Autodesk Inventor part; units mm, degrees
ref_plane "YZ Plane" through (0, 0, 0) normal (1, 0, 0) x (0, 1, 0)
ref_plane "XZ Plane" through (0, 0, 0) normal (0, 1, 0) x (-1, 0, 0)
ref_plane "XY Plane" through (0, 0, 0) normal (0, 0, 1) x (1, 0, 0)
sketch "Skizze1" plane through (0, 0, 0) normal (0, 1, 0) x (-1, 0, 0)
  line L0 (87.5, -100) -> (-87.5, -100)
  line L1 (-87.5, -100) -> (-87.5, 100)
  line L2 (-87.5, 100) -> (87.5, 100)
  line L3 (87.5, 100) -> (87.5, -100)
  line L4 (0, -140) -> (0, 140)
  line L5 (122.5, 0) -> (-122.5, 0)
  point P0 (0, 0)
  dimension "d0" = 175
  dimension "d1" = 200
extrude "Extrusion1" add sketch "Skizze1" along normal blind 2
sketch "Skizze2" plane through (0, 2, 0) normal (0, 1, 0) x (1, 0, 0)
  circle A0 centre (54.5, 95) radius 1.6
  circle A1 centre (-82.5, 95) radius 1.6
  line L0 (0, 140) -> (0, -140)
  line L1 (122.5, 0) -> (-122.5, 0)
  line L2 (87.5, 100) -> (-87.5, 100)
  circle A2 centre (54.5, -95) radius 1.6
  circle A3 centre (-82.5, -95) radius 1.6
  line L3 (-87.5, 100) -> (-87.5, -100)
  line L4 (87.5, -100) -> (87.5, 100)
  point P0 (0, 0)
  dimension "d4" = 3.2
  dimension "d5" = 3.2
  dimension "d7" = 5
  dimension "d9" = 5
  dimension "d55" = 5
  dimension "d56" = 33
extrude "Extrusion2" cut sketch "Skizze2" against normal up to surface (2 mm away) contours A0 | A1 | A2 | A3
sketch "Skizze3" plane through (0, 2, 0) normal (0, 1, 0) x (1, 0, 0)
  line L0 (0, 140) -> (0, -140)
  line L1 (122.5, 0) -> (-122.5, 0)
  line L2 (-87.5, -100) -> (87.5, -100)
  line L3 (-87.5, 100) -> (-87.5, -100)
  circle A0 centre (64.5, -89.5) radius 1.6
  line L4 (87.5, -100) -> (87.5, 100)
  circle A1 centre (64.5, -25.5) radius 1.6
  circle A2 centre (64.5, 25.5) radius 1.6
  line L5 (87.5, 100) -> (-87.5, 100)
  circle A3 centre (64.5, 89.5) radius 1.6
  circle A4 centre (27.5, -23) radius 1.6
  circle A5 centre (27.5, 23) radius 1.6
  point P0 (0, 0)
  dimension "d35" = 3.2
  dimension "d36" = 10.5
  dimension "d37" = 23
  dimension "d38" = 3.2
  dimension "d39" = 74.5
  dimension "d40" = 23
  dimension "d41" = 3.2
  dimension "d42" = 23
  dimension "d43" = 74.5
  dimension "d44" = 3.2
  dimension "d45" = 23
  dimension "d46" = 10.5
  dimension "d47" = 3.2
  dimension "d48" = 60
  dimension "d49" = 77
  dimension "d50" = 3.2
  dimension "d51" = 60
  dimension "d52" = 77
extrude "Extrusion3" cut sketch "Skizze3" against normal up to surface (2 mm away) contours A0 | A1 | A2 | A3 | A4 | A5
sketch "Skizze4" plane through (0, 2, 0) normal (0, 1, 0) x (1, 0, 0)
  line L0 (-47.5, -36.6) -> (5.84, -36.6)
  line L1 (5.84, -36.6) -> (5.84, 65)
  line L2 (5.84, 65) -> (-47.5, 65)
  line L3 (-47.5, 65) -> (-47.5, -36.6)
  line L4 (122.5, 0) -> (-122.5, 0)
  line L5 (-87.5, 100) -> (-87.5, -100)
  circle A0 centre (3.3, 49.76) radius 3.5
  circle A1 centre (3.3, -25.17) radius 3.5
  circle A2 centre (-44.96, -31.52) radius 3.5
  circle A3 centre (-44.96, 51.03) radius 3.5
  line L6 (87.5, 100) -> (-87.5, 100)
  point P0 (0, 0)
  point P1 (-15.83, 0)
  dimension "d57" = 53.34
  dimension "d58" = 101.6
  dimension "d59" = 40
  dimension "d60" = 7
  dimension "d61" = 86.36
  dimension "d62" = 50.8
  dimension "d63" = 7
  dimension "d64" = 90.17
  dimension "d65" = 50.8
  dimension "d66" = 7
  dimension "d67" = 96.52
  dimension "d68" = 50.8
  dimension "d69" = 7
  dimension "d70" = 87.63
  dimension "d71" = 50.8
  dimension "d140" = 35
extrude "Extrusion4" add sketch "Skizze4" along normal blind 7 contours A2 L3 | L3 A2 | A1 L1 | L1 A1 | A3 L3 | L3 A3 | A0 L1 | L1 A0
sketch "Skizze5" plane through (3.3, 9, -49.76) normal (0, 1, 0) x (1, 0, 0)
  circle A0 centre (0, 0) radius 3.5
  circle A1 centre (-48.26, 1.27) radius 3.5
  circle A2 centre (-48.26, -81.28) radius 3.5
  circle A3 centre (0, -74.93) radius 3.5
  circle A4 centre (0, 0) radius 2
  circle A5 centre (0, -74.93) radius 2
  circle A6 centre (-48.26, 1.27) radius 2
  circle A7 centre (-48.26, -81.28) radius 2
  point P0 (-3.3, -49.76)
  dimension "d74" = 4
  dimension "d75" = 4
  dimension "d76" = 4
  dimension "d77" = 4
extrude "Extrusion5" cut sketch "Skizze5" against normal blind 5 contours A4 | A5 | A6 | A7
sketch "Skizze6" plane through (0, 2, 0) normal (0, 1, 0) x (1, 0, 0)
  circle A0 centre (72.5, 35) radius 1.6
  circle A1 centre (72.5, 52) radius 1.6
  line L0 (87.5, -100) -> (87.5, 100)
  line L1 (-122.5, 0) -> (122.5, 0)
  circle A2 centre (37.5, 35) radius 1.6
  circle A3 centre (37.5, 52) radius 1.6
  point P0 (0, 0)
  dimension "d80" = 3.2
  dimension "d81" = 3.2
  dimension "d82" = 15
  dimension "d83" = 15
  dimension "d84" = 35
  dimension "d85" = 17
  dimension "d88" = 3.2
  dimension "d89" = 3.2
  dimension "d90" = 50
  dimension "d91" = 50
  dimension "d92" = 35
  dimension "d94" = 17
extrude "Extrusion6" cut sketch "Skizze6" against normal up to surface (2 mm away)
sketch "Skizze7" plane through (0, 2, 0) normal (0, 1, 0) x (1, 0, 0)
  line L0 (16, -90.8) -> (9, -90.8)
  line L1 (9, -90.8) -> (9, -97.8)
  line L2 (9, -97.8) -> (16, -97.8)
  line L3 (16, -97.8) -> (16, -90.8)
  line L4 (-87.5, 100) -> (-87.5, -100)
  line L5 (-87.5, -100) -> (87.5, -100)
  line L6 (122.5, 0) -> (-122.5, 0)
  line L7 (16, 90.8) -> (9, 90.8)
  line L8 (9, 90.8) -> (9, 97.8)
  line L9 (9, 97.8) -> (16, 97.8)
  line L10 (16, 97.8) -> (16, 90.8)
  point P0 (0, 0)
  dimension "d95" = 103.5
  dimension "d96" = 7
  dimension "d97" = 7
  dimension "d98" = 2.2
extrude "Extrusion7" add sketch "Skizze7" along normal blind 9
sketch "Skizze8" plane through (9, 2, 97.8) normal (0, 0, 1) x (1, 0, 0)
  circle A0 centre (3.5, 5) radius 2
  line L0 (7, 0) -> (0, 0)
  line L1 (7, 0) -> (7, 9)
  point P0 (-9, -2)
  dimension "d101" = 4
  dimension "d102" = 5
  dimension "d103" = 3.5
extrude "Extrusion8" cut sketch "Skizze8" against normal blind 5
sketch "Skizze9" plane through (16, 2, -97.8) normal (0, 0, -1) x (-1, 0, 0)
  circle A0 centre (3.5, 5) radius 2
  line L0 (7, 0) -> (7, 9)
  line L1 (7, 0) -> (0, 0)
  point P0 (16, -2)
  dimension "d107" = 4
  dimension "d108" = 3.5
  dimension "d109" = 5
extrude "Extrusion9" cut sketch "Skizze9" against normal blind 5
fillet "Rundung1" radius 3.5 4 edges at (16, 11, -94.3) (9, 11, -94.3) (9, 11, 94.3) (16, 11, 94.3)
sketch "Skizze10" plane through (0, 2, 0) normal (0, 1, 0) x (1, 0, 0)
  line L0 (-59.5, 20) -> (-79.5, 20)
  line L1 (-79.5, 20) -> (-79.5, -20)
  line L2 (-79.5, -20) -> (-59.5, -20)
  line L3 (-59.5, -20) -> (-59.5, 20)
  line L4 (122.5, 0) -> (-122.5, 0)
  line L5 (-87.5, 100) -> (-87.5, -100)
  point P0 (0, 0)
  dimension "d113" = 20
  dimension "d114" = 40
  dimension "d115" = 8
extrude "Extrusion10" cut sketch "Skizze10" against normal up to surface (2 mm away)
sketch "Skizze11" plane through (0, 2, 0) normal (0, 1, 0) x (1, 0, 0)
  circle A0 centre (-1.5, -51) radius 3.5
  circle A1 centre (-1.5, -87) radius 3.5
  circle A2 centre (-57.5, -51) radius 3.5
  circle A3 centre (-57.5, -87) radius 3.5
  line L0 (-87.5, 100) -> (-87.5, -100)
  line L1 (87.5, 100) -> (-87.5, 100)
  line L2 (-87.5, -100) -> (87.5, -100)
  point P0 (0, 0)
  dimension "d118" = 7
  dimension "d119" = 7
  dimension "d120" = 7
  dimension "d121" = 7
  dimension "d122" = 30
  dimension "d123" = 30
  dimension "d126" = 56
  dimension "d127" = 36
  dimension "d128" = 56
  dimension "d129" = 36
  dimension "d138" = 13
  dimension "d139" = 13
extrude "Extrusion11" add sketch "Skizze11" along normal blind 7
sketch "Skizze12" plane through (-1.5, 9, 51) normal (0, 1, 0) x (1, 0, 0)
  circle A0 centre (0, 0) radius 3.5
  circle A1 centre (0, -36) radius 3.5
  circle A2 centre (-56, -36) radius 3.5
  circle A3 centre (-56, 0) radius 3.5
  circle A4 centre (0, 0) radius 2.15
  circle A5 centre (0, -36) radius 2.15
  circle A6 centre (-56, 0) radius 2.15
  circle A7 centre (-56, -36) radius 2.15
  point P0 (1.5, 51)
  dimension "d132" = 4.3
  dimension "d133" = 4.3
  dimension "d134" = 4.3
  dimension "d135" = 4.3
extrude "Extrusion12" cut sketch "Skizze12" against normal blind 6 contours A4 | A5 | A6 | A7
equation "\"d10\" = d6"
equation "\"d53\" = d48"
properties part number "_3D-Druck"
Verification items for the finished model (mm, model axes). A direction names the side the tool comes from. Coordinates: 2 decimals unless noted, no trailing zeros. Order: outer loops, then holes, each group sorted by start corner. A loop starts at its lowest first (then second) coordinate and runs counter-clockwise, first axis right, second up.
Item 1: Material ranges on L1, parallel to Z at x = 64.5, y = 0.5; L2, parallel to Z at x = -82.5, y = 0.8; L3, parallel to X at y = 0.8, z = 95, recorded low to high.
Filled in:
L1: z = -100 to -91.1, -87.9 to -27.1, -23.9 to 23.9, 27.1 to 87.9, 91.1 to 100
L2: z = -100 to -96.6, -93.4 to 93.4, 96.6 to 100
L3: x = -87.5 to -84.1, -80.9 to 52.9, 56.1 to 87.5
Item 2: Depth check by flat-ended pin: pin 1 (2.5 mm diameter, centred on x = 64.5, z = 89.5, fed in from -Y) (3 decimals); pin 2 (2 mm diameter, centred on x = 3.5, z = 25, fed in from +Y); pin 3 (3 mm diameter, centred on x = 12, y = 6.5, fed in from +Z); pin 4 (3 mm diameter, centred on x = 11, z = -19, fed in from +Y). Enter the tip coordinate at first touch or a pass-through.
Filled in:
pin 1: passes through
pin 2: stops at y = 4
pin 3: stops at z = 97.8
pin 4: stops at y = 2
Item 3: Section check B-B, the plane z = 64. Enter the section's corners in (x, y).
Filled in:
outline: (-87.5, 0) - (87.5, 0) - (87.5, 2) - (-87.5, 2) - close
Item 4: Section check A-A, the plane x = 50.5. Enter the section's corners in (y, z), then the cut area to 3 significant figures.
Filled in:
outline: (0, -100) - (2, -100) - (2, 100) - (0, 100) - close
area: 400 mm2
Item 5: Access from +Z, -Z, +X, -X, +Y, -Y to the whole of each face (thin tool, end or side, straight path). Record for faces 5 (the face through (16, 5, 94)), 6 (the face through (-0.34, 6.04, 49.19)), 7 (the face through (0, 9, 49)), 8 (the face through (1, 0, 1)), 9 (the face through (12, 4, -97.8)).
Filled in:
face 5: +Z, -Z, +X, +Y
face 6: +Y
face 7: +Z, -Z, +X, -X, +Y
face 8: +Z, -Z, +X, -X, -Y
face 9: -Z, +X, -X, +Y
Item 6: Release check for a two-part mould opening along Y. For faces 1 (the face through (12, 7, 92.8)), 2 (the face through (13, 6, -90.8)), 3 (the face through (13, 7, -92.8)), 4 (the face through (-56, 9, 85)) record: +Y half, -Y half, draft (parallel to the pull), parting line (faces both ways), or undercut.
Filled in:
face 1: undercut
face 2: draft
face 3: undercut
face 4: +Y half
